```python
from build123d import *

# Parameters (mm, degrees)
F0_W     = 500
F0_H     = 25
F1_DEPTH = 15
F2_R     = 75
F3_DEPTH = 5
F4_W     = 7.5
F4_H     = 7.5
F5_DEPTH = 12.5


with BuildPart() as f1:
    # F0 (on Top) → F1 (new body)
    with BuildSketch(Plane.XY):
        with Locations((-250, 0)):
            Rectangle(F0_W, F0_H)
    extrude(amount=-F1_DEPTH)

    # F2 (on Top) → F3 (join)
    with BuildSketch(Plane.XY):
        with Locations((-400, 0)):
            Circle(F2_R)
    extrude(amount=F3_DEPTH)

    # F4 (on Front) → F5 (cut, symmetric)
    with BuildSketch(Plane.XZ):
        with Locations((-316.25, -11.25)):
            Rectangle(F4_W, F4_H)
    extrude(amount=F5_DEPTH, both=True, mode=Mode.SUBTRACT)


solid = f1.part
```
For this review, take the finished solid that the model builds, in its own axes (mm). A direction names the side the tool comes from. Round coordinates to 2 decimals unless told otherwise and drop trailing zeros. Write each loop counter-clockwise with the first axis right and the second up, starting at its lowest first coordinate (ties: lowest second). Pieces come first, ordered by that corner, then holes. Notation, with made-up numbers: (62, 6.25) -> (84, 6.25) arc R21 ccw to (84, 24.25) -> close; hole circle Ø11 at (80, 64). An arc over 180 degrees is marked (long way). One line per question, with ' | ' between items. Start each with the question number.
(1) For line 1 along Y through (x, z) = (-259.5, -11.25); line 2 along Z through (x, y) = (-317, -1); line 3 along Z through (x, y) = (-353.5, -29), list the stretches that pass through material, from the lowest coordinate up. Write a range as from..to.
(2) Add section B-B, the plane x = -400. Write out the cut boundary in (y, z).
(3) Mouldability with a two-part tool opening along X and no side actions: class faces 5 (the face through (0, 0, -7)), 6 (the face through (-401, 1, 5)), 7 (the face through (-500, 0, -7)) as released by +X, released by -X, zero draft, split by the parting line, or undercut.
(4) Add section A-A, the plane z = -12. Write out the cut boundary in (x, y).
(5) Add section D-D, the plane x = -347.5. Write out the cut boundary in (y, z), plus the area to 3 significant figures.
(6) Add section C-C, the plane y = 0. Write out the cut boundary in (x, z).
(7) Insertion check: P1, Ø20, axis at x = -189, y = -1.5, coming from the +Z side; P2, Ø4.5, axis at x = -173, z = -8.5, coming from the -Y side; P3, Ø4, axis at x = -317.5, z = -4.5, coming from the +Y side. Each pin has a flat end and moves straight along its axis. Give the tip position at first contact, or say it passes through.
(8) Tool access review of faces 1 (the face through (-253, -12.5, -7)), 2 (the face through (-165, 0, 0)), 3 (the face through (-411, 0, -15)), 4 (the face through (-253, 12.5, -7)): name each direction out of +Z, -Z, +X, -X, +Y, -Y from which nothing blocks a thin tool from reaching the whole face with its end or side.
Answer list:
1) line 1: -12.5..12.5 | line 2: -7.5..0 | line 3: 0..5
2) outline: (-75, 0) -> (-12.5, 0) -> (-12.5, -15) -> (12.5, -15) -> (12.5, 0) -> (75, 0) -> (75, 5) -> (-75, 5) -> close
3) face 5: released by +X | face 6: zero draft | face 7: released by -X
4) outline: (-500, -12.5) -> (-320, -12.5) -> (-320, 12.5) -> (-500, 12.5) -> close; (-312.5, -12.5) -> (0, -12.5) -> (0, 12.5) -> (-312.5, 12.5) -> close
5) outline: (-53.56, 0) -> (-12.5, 0) -> (-12.5, -15) -> (12.5, -15) -> (12.5, 0) -> (53.56, 0) -> (53.56, 5) -> (-53.56, 5) -> close | area: 911 mm²
6) outline: (-500, -15) -> (-320, -15) -> (-320, -7.5) -> (-312.5, -7.5) -> (-312.5, -15) -> (0, -15) -> (0, 0) -> (-325, 0) -> (-325, 5) -> (-475, 5) -> (-475, 0) -> (-500, 0) -> close
7) P1: z = 0 | P2: y = -12.5 | P3: y = 12.5
8) face 1: -Z, +X, -X, -Y | face 2: +Z, +X, +Y, -Y | face 3: -Z, +X, -X, +Y, -Y | face 4: -Z, +X, -X, +Y
